Here's the drawing with two shaded views (mm, measured from the low corner). I have some questions. A direction names the side the tool comes from. Coordinates: 2 decimals unless noted, no trailing zeros. Write each loop counter-clockwise with the first axis right and the second up, starting at its lowest first coordinate (ties: lowest second). Pieces come first, ordered by that corner, then holes. Notation, with made-up numbers: M 12,89.25 L 18,89.25 A12 cw 18,109.25 Z; hole C 18,74 d4. An arc over 180 degrees is marked long. Answer as CSV lines item,"result". Start each with the question number.
Item 1: Suppose I cut it at B-B, the plane y = 2. Write out the boundary of the cut face in (x, z).
Item 2: On a 3-axis mill with a long thin cutter (end or side, diameter ignored), from which of +Z, -Z, +X, -X, +Y, -Y can I reach the whole of each face in a straight line? I mean the marked faces 1 and 2. Say none if no direction works.
Item 3: If I drill on line 1 along Y through (x, z) = (5.05, 3.2); line 2 along Z through (x, y) = (2.8, 14.75); line 3 along X through (y, z) = (11.5, 3.15) (1 decimal), over which ranges is the centre line in solid material (lowest first)? Write a range as [from, to].
Item 4: Suppose I cut it at C-C, the plane x = 3.7. Write out the boundary of the cut face in (y, z) (1 decimal).
Item 5: I'm going to push flat-ended pins straight in: P1, Ø1, axis at y = 5, z = 2, coming from the -X side; P2, Ø2, axis at x = 3, z = 3.5, coming from the -Y side; P3, Ø0.8, axis at x = 2.5, z = 2.5, coming from the -Y side; P4, Ø1, axis at x = 4, y = 9.5, coming from the -Z side. Where does each tip first touch, or does it pass through?
Item 6: Suppose I cut it at D-D, the plane y = 5.75. Write out the boundary of the cut face in (x, z).
Item 7: Suppose I cut it at A-A, the plane z = 2.75. Write out the boundary of the cut face in (x, y).
Item 8: We'd pull the mould along Z, two halves only. Please class the marked faces 3, 4 and 5: +Z half, -Z half, draft (parallel to the pull), parting line (faces both ways), or undercut.
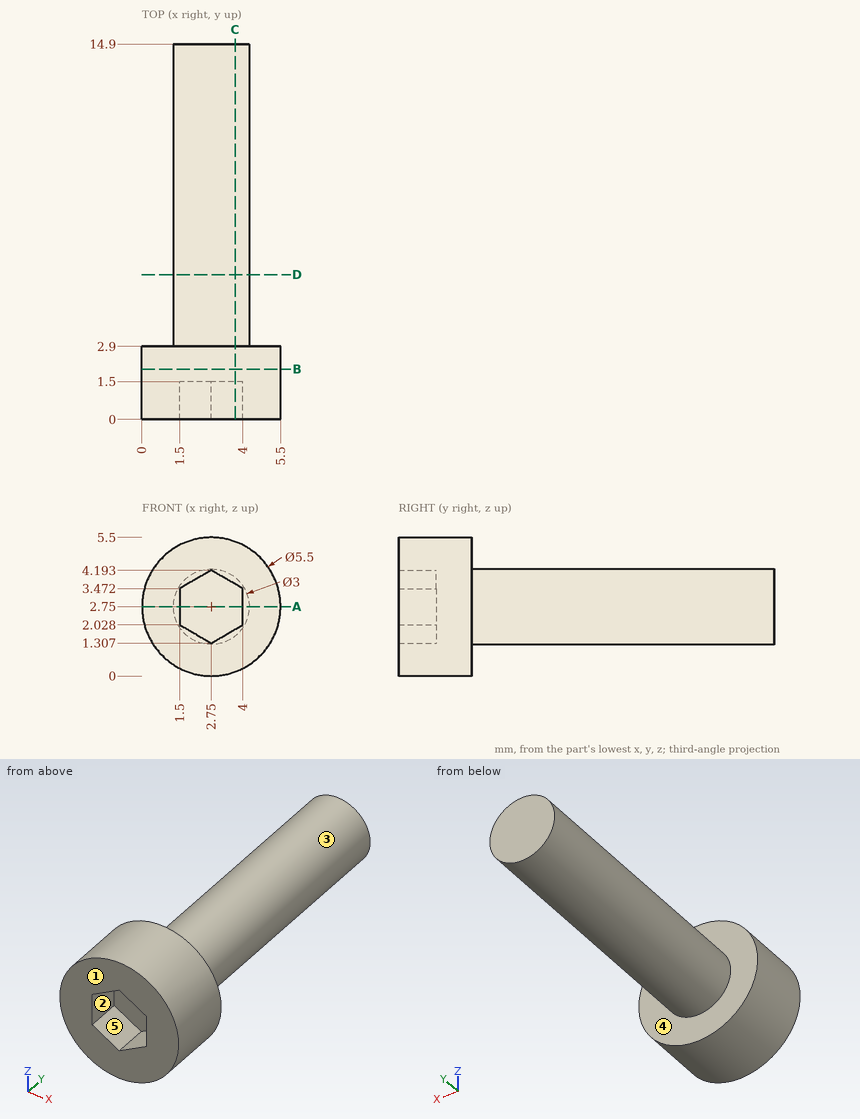
Ans:
1,outline,"C 2.75,2.75 d5.5"
2,face 1,"+Z, -Z, +X, -X, -Y"
2,face 2,"-Y"
3,line 1,"y = [0, 2.9]"
3,line 2,"z = [1.25, 4.25]"
3,line 3,"x = [1.3, 4.2]"
4,outline,"M 0,0.2 L 2.9,0.2 L 2.9,1.6 L 14.9,1.6 L 14.9,3.9 L 2.9,3.9 L 2.9,5.3 L 0,5.3 L 0,3.6 L 1.5,3.6 L 1.5,1.9 L 0,1.9 Z"
5,P1,"stops at x = 1.27"
5,P2,"stops at y = 0"
5,P3,"stops at y = 1.5"
5,P4,"stops at z = 1.45"
6,outline,"C 2.75,2.75 d3"
7,outline,"M 0,0 L 1.5,0 L 1.5,1.5 L 4,1.5 L 4,0 L 5.5,0 L 5.5,2.9 L 4.25,2.9 L 4.25,14.9 L 1.25,14.9 L 1.25,2.9 L 0,2.9 Z"
8,face 3,"parting line"
8,face 4,"draft"
8,face 5,"undercut"
